For this review, take the finished solid that the model builds, in its own axes (mm). Face numbers are marked on the shaded views. A direction names the side the tool comes from. Round coordinates to 2 decimals unless told otherwise and drop trailing zeros. Write each loop counter-clockwise with the first axis right and the second up, starting at its lowest first coordinate (ties: lowest second). Pieces come first, ordered by that corner, then holes. Notation, with made-up numbers: (80, 72) - (84, 72) arc R21 ccw to (84, 85) - close; hole circle Ø10 at (-3, 19.5). An arc over 180 degrees is marked (long way). One line per item, written item: value. Start each with the question number.
Q1. Add section B-B on x = 13.9. Write out the cut boundary in (y, z).
Q2. Mouldability with a two-part tool opening along X and no side actions: class the marked faces 1, 2 and 3 as +X half, -X half, draft (parallel to the pull), parting line (faces both ways), or undercut.
Q3. For probe 1 along X at (y, z) = (0.45, 5.5); probe 2 along Y at (x, z) = (-26.5, 9.65); probe 3 along X at (y, z) = (2, 5), list the stretches that pass through material, from the lowest coordinate up.
Q4. Add section D-D on y = -3. Write out the cut boundary in (x, z).
Q5. Clearance check with flat-ended pins moving along their axes: pin 1 Ø1.5 at (y, z) = (2.5, 3) entering from +X; pin 2 Ø9.5 at (y, z) = (-5, 6.5) entering from +X; pin 3 Ø9.5 at (x, z) = (-7.5, 4.5) entering from -Y; pin 4 Ø3 at (x, y) = (-1, 3) entering from +Z. State where each tip first meets the part, or that it passes through.
Q6. Add section A-A on z = 9.75. Write out the cut boundary in (x, y).
Q7. Add section C-C on z = 5.5. Write out the cut boundary in (x, y), and give its area (3 significant figures).
Q8. Tool access review of the marked faces 4, 5, 6 and 7: name each direction out of +Z, -Z, +X, -X, +Y, -Y from which nothing blocks a thin tool from reaching the whole face with its end or side.
```python
from build123d import *

# Parameters (mm, degrees)
RESSALTO_EXTRUS_O1_DEPTH   = 4
FURO_DE_DI_METRO_2_0_2_1_D = 2
RESSALTO_EXTRUS_O2_DEPTH   = 4
FURO_COM_FOLGA_DE_M41_D    = 4.5
ESBO_O6_W                  = 32
ESBO_O6_H                  = 12
CORTE_EXTRUS_O1_DEPTH      = 3


with BuildPart() as part:
    # Esboço1 → Ressalto-extrusão1 (new body)
    with BuildSketch(Plane(origin=(0, 0, 0), x_dir=(1, 0, 0), z_dir=(0, 1, 0))):
        Polygon((-19.5, 4), (-19.5, -12), (-11.5, -12), (-11.5, 0), (11.5, 0), (11.5, -12), (19.5, -12), (19.5, 4), align=None)
    extrude(amount=RESSALTO_EXTRUS_O1_DEPTH)

    # Furo de diâmetro Ø2.0 (2)1 (through all)
    with Locations(Plane(origin=(-13.9, 4, 5.5), x_dir=(0, 0, 1), z_dir=(0, 1, 0))):
        with Locations((0, 0), (0, 27.8)):
            Hole(FURO_DE_DI_METRO_2_0_2_1_D / 2)

    # Esboço4 → Ressalto-extrusão2 (add)
    with BuildSketch(Plane.XY.offset(12)):
        Polygon((31.5, -16), (31.5, -6), (19.5, -6), (19.5, 4), (11.5, 4), (11.5, -16), align=None)
        Polygon((-19.5, 4), (-11.5, 4), (-11.5, -16), (-31.5, -16), (-31.5, -6), (-19.5, -6), align=None)
    extrude(amount=-RESSALTO_EXTRUS_O2_DEPTH)

    # Furo com folga de M41 (through all)
    with Locations(Plane(origin=(-26.5, -11, 12), x_dir=(1, 0, 0), z_dir=(0, 0, 1))):
        with Locations((0, 0), (53, 0)):
            Hole(FURO_COM_FOLGA_DE_M41_D / 2)

    # Esboço6 → Corte-extrusão1 (cut)
    with BuildSketch(Plane(origin=(0, 4, 0), x_dir=(1, 0, 0), z_dir=(0, 1, 0))):
        with Locations((0, -6)):
            Rectangle(ESBO_O6_W, ESBO_O6_H)
    extrude(amount=-CORTE_EXTRUS_O1_DEPTH, mode=Mode.SUBTRACT)


solid = part.part
```
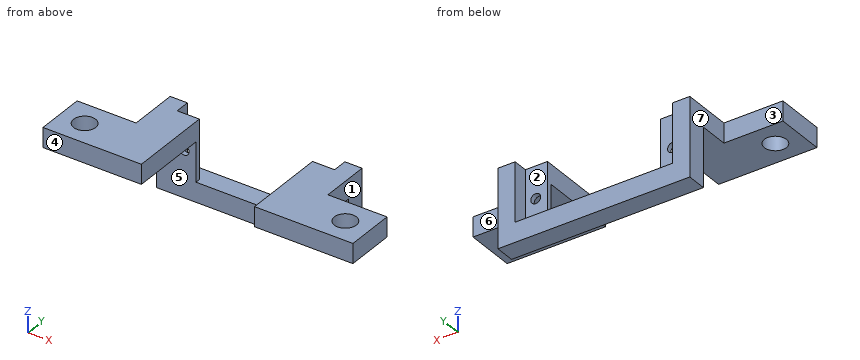
Result set:
1. outline: (-16, 8) - (0, 8) - (0, 6.5) - (1, 6.5) - (1, 12) - (-16, 12) - close; (0, -4) - (4, -4) - (4, 0) - (1, 0) - (1, 4.5) - (0, 4.5) - close
2. face 1: +X half
2. face 2: undercut
2. face 3: draft
3. probe 1: x = -19.5 to -14.9, -12.9 to -11.5, 11.5 to 12.9, 14.9 to 19.5
3. probe 2: y = -16 to -13.25, -8.75 to -6
3. probe 3: x = -19.5 to -16, 16 to 19.5
4. outline: (-19.5, 8) - (-11.5, 8) - (-11.5, 12) - (-19.5, 12) - close; (11.5, 8) - (19.5, 8) - (19.5, 12) - (11.5, 12) - close
5. pin 1: stops at x = 19.5
5. pin 2: stops at x = 31.5
5. pin 3: stops at y = 0
5. pin 4: stops at z = 0
6. outline: (-31.5, -16) - (-11.5, -16) - (-11.5, 1) - (-16, 1) - (-16, 4) - (-19.5, 4) - (-19.5, -6) - (-31.5, -6) - close; (11.5, -16) - (31.5, -16) - (31.5, -6) - (19.5, -6) - (19.5, 4) - (16, 4) - (16, 1) - (11.5, 1) - close; hole circle Ø4.5 at (-26.5, -11); hole circle Ø4.5 at (26.5, -11)
7. outline: (-19.5, 0) - (-14.9, 0) - (-14.9, 1) - (-16, 1) - (-16, 4) - (-19.5, 4) - close; (-12.9, 0) - (-11.5, 0) - (-11.5, 1) - (-12.9, 1) - close; (11.5, 0) - (12.9, 0) - (12.9, 1) - (11.5, 1) - close; (14.9, 0) - (19.5, 0) - (19.5, 4) - (16, 4) - (16, 1) - (14.9, 1) - close
7. area: 33.0 mm^2
8. face 4: +Z, -Z, +X, -X, -Y
8. face 5: -Z, +X, -X, -Y
8. face 6: +Z, -Z, +X, +Y
8. face 7: +Z, -Z, -X, +Y
